Part model, mm, in its own coordinate system. A direction names the side the tool comes from. Round coordinates to 2 decimals unless told otherwise and drop trailing zeros. Loops run counter-clockwise (first coordinate to the right, second up) from the corner with the lowest first, then second, coordinate; pieces in that order, holes last.
1) Band-saw the part on A-A, the plane z = 9. State how many separate pieces and enclosed holes the cut face has, then the cut area to 3 significant figures.
2) 3-axis set-ups, long thin cutter, end or side, ignore diameter. For faces 1 (the cylindrical face through (74.01, 21.64, 26.28)), 2 (the flat face through (73, -1, 26)): which of +Z, -Z, +X, -X, +Y, -Y reach the whole face in a straight line?
3) Band-saw the part on B-B, the plane x = -25.5. Write the cut outline in (y, z).
4) Drop flat-ended pins along their axis: P1, Ø2, axis at x = 3, y = -48.5, coming from the +Z side; P2, Ø5, axis at x = 18.5, y = 9, coming from the +Z side; P3, Ø2, axis at y = 59, z = 39, coming from the +X side. Give the stop position or say it passes through.
5) Mould opens along X. For faces 3 (the flat face through (1, 60, 25)), 4 (the flat face through (75, -1, 25)), 5 (the cylindrical face through (56.845, -48.074, 4.465)) say: +X half, -X half, draft (parallel to the pull), parting line (faces both ways), or undercut.
6) Band-saw the part on C-C, the plane y = -11.5. Write the cut outline in (x, z), then the cut area to 3 significant figures.
7) Probe line 1 (Y direction, x = 46.54, z = 4.35) (3 decimals); line 2 (X direction, y = 39, z = 47.5); line 3 (Y direction, x = -37.5, z = 28.5). List the from-to ranges inside material, lowest first.
from build123d import *

# Parameters (mm, degrees)
F1_DEPTH  = 50
F2_T      = -2
F3_R      = 2.5
F3_R_2    = 1.25
F4_DEPTH  = 30
F5_W      = 9
F5_H      = 5
F6_DEPTH  = 2
F8_R      = 4.25
F8_W      = 13
F8_H      = 20
F9_DEPTH  = 2
F10_R     = 2.5
F10_R_2   = 1.25
F11_DEPTH = 5


with BuildPart() as f1:
    # F0 (on Top) → F1 (new body)
    with BuildSketch(Plane.XY):
        with BuildLine():
            Line((60, 60), (-60, 60))
            ThreePointArc((-60, 60), (-70.606602, 55.606602), (-75, 45))
            Line((-75, 45), (-75, -45))
            ThreePointArc((-75, -45), (-70.606602, -55.606602), (-60, -60))
            Line((-60, -60), (60, -60))
            ThreePointArc((60, -60), (70.606602, -55.606602), (75, -45))
            Line((75, -45), (75, 45))
            ThreePointArc((75, 45), (70.606602, 55.606602), (60, 60))
        make_face()
    extrude(amount=F1_DEPTH)

    # F2
    f2_openings = [f1.faces().sort_by_distance(p)[0] for p in [
        (0, 0, 50),
    ]]
    offset(amount=F2_T, openings=f2_openings)

    # F3 (on face) → F4 (join)
    with BuildSketch(Plane.XY.offset(2)):
        with Locations((-6.825, 54.825)):
            Circle(F3_R)
        with Locations((-6.825, 54.825)):
            Circle(F3_R_2, mode=Mode.SUBTRACT)
        with Locations((-6.825, 11.175)):
            Circle(F3_R)
        with Locations((-6.825, 11.175)):
            Circle(F3_R_2, mode=Mode.SUBTRACT)
        with Locations((56.825, 54.825)):
            Circle(F3_R)
        with Locations((56.825, 54.825)):
            Circle(F3_R_2, mode=Mode.SUBTRACT)
        with Locations((56.825, 11.175)):
            Circle(F3_R)
        with Locations((56.825, 11.175)):
            Circle(F3_R_2, mode=Mode.SUBTRACT)
    extrude(amount=F4_DEPTH)

    # F5 (on face) → F6 (cut, through all)
    with BuildSketch(Plane(origin=(0, 60, 0), x_dir=(-1, 0, 0), z_dir=(0, 1, 0))):
        with Locations((-6, 39)):
            Rectangle(F5_W, F5_H)
    extrude(amount=-F6_DEPTH, mode=Mode.SUBTRACT)

    # F8 (on face) → F9 (cut, through all)
    with BuildSketch(Plane.YZ.offset(75)):
        with Locations((17.588826, 25)):
            Circle(F8_R)
        with Locations((37.588826, 25)):
            Rectangle(F8_W, F8_H)
    extrude(amount=-F9_DEPTH, mode=Mode.SUBTRACT)

    # F10 (on face) → F11 (join)
    with BuildSketch(Plane.XY.offset(2)):
        with Locations((-4.46, -48.825)):
            Circle(F10_R)
        with Locations((-4.46, -48.825)):
            Circle(F10_R_2, mode=Mode.SUBTRACT)
        with Locations((3.46, -48.825)):
            Circle(F10_R)
        with Locations((3.46, -48.825)):
            Circle(F10_R_2, mode=Mode.SUBTRACT)
        with Locations((12.54, -48.825)):
            Circle(F10_R)
        with Locations((12.54, -48.825)):
            Circle(F10_R_2, mode=Mode.SUBTRACT)
        with Locations((20.46, -48.825)):
            Circle(F10_R)
        with Locations((20.46, -48.825)):
            Circle(F10_R_2, mode=Mode.SUBTRACT)
        with Locations((29.54, -48.825)):
            Circle(F10_R)
        with Locations((29.54, -48.825)):
            Circle(F10_R_2, mode=Mode.SUBTRACT)
        with Locations((37.46, -48.825)):
            Circle(F10_R)
        with Locations((37.46, -48.825)):
            Circle(F10_R_2, mode=Mode.SUBTRACT)
        with Locations((46.54, -48.825)):
            Circle(F10_R)
        with Locations((46.54, -48.825)):
            Circle(F10_R_2, mode=Mode.SUBTRACT)
        with Locations((54.46, -48.825)):
            Circle(F10_R)
        with Locations((54.46, -48.825)):
            Circle(F10_R_2, mode=Mode.SUBTRACT)
    extrude(amount=F11_DEPTH)


solid = f1.part
Reported:
1. separate pieces: 5
1. enclosed holes: 5
1. area: 1,070 mm2
2. face 1: +X
2. face 2: +Z
3. outline: (-60, 0) - (60, 0) - (60, 50) - (58, 50) - (58, 2) - (-58, 2) - (-58, 50) - (-60, 50) - close
4. P1: stops at z = 7
4. P2: stops at z = 2
4. P3: stops at x = 67.48
5. face 3: draft
5. face 4: +X half
5. face 5: undercut
6. outline: (-75, 0) - (75, 0) - (75, 50) - (73, 50) - (73, 2) - (-73, 2) - (-73, 50) - (-75, 50) - close
6. area: 492 mm2
7. line 1: y = -60 to -58, -51.325 to -50.075, -47.575 to -46.325, 58 to 60
7. line 2: x = -75 to -73, 73 to 75
7. line 3: y = -60 to -58, 58 to 60
